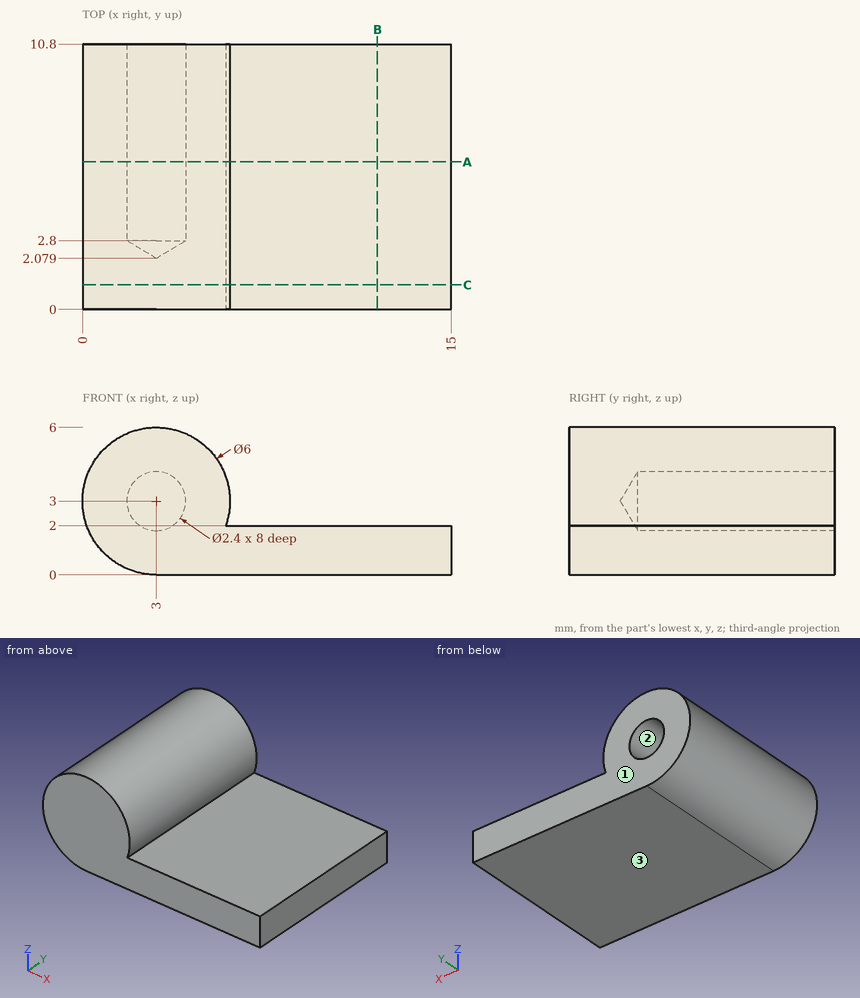
Design review of the part shown in the three views and the two pictorial views. Dimensions are in mm from the part's minimum x, y and z. Round coordinates to 2 decimals unless told otherwise and drop trailing zeros. Order: outer loops, then holes, each group sorted by start corner. A loop starts at its lowest first (then second) coordinate and runs counter-clockwise, first axis right, second up. Notation, with made-up numbers: (-19, -34.5) -> (17, -34.5) arc R21 cw to (17, -29.5) -> close; hole circle Ø9 at (14, 39). An arc over 180 degrees is marked (long way). Write item = value, one per line. Start each with the question number.
1) Take a section at B-B on x = 12. State the section outline as (y, z) points.
2) The part is to be moulded in two halves that separate along Z. For the marked faces 1, 2 and 3, say which applies: +Z half, -Z half, draft (parallel to the pull), parting line (faces both ways), or undercut.
3) To check wall thickness, follow line 1 (X direction, y = 9, z = 3); line 2 (Z direction, x = 13.25, y = 1); line 3 (Z direction, x = 3.5, y = 2.5). State the ranges of each line that lie inside material, in increasing order. Write a range as from..to.
4) Take a section at A-A on y = 6. State the section outline as (x, z) points, plus the area to 3 significant figures.
5) Take a section at C-C on y = 1. State the section outline as (x, z) points, plus the area to 4 significant figures.
6) Insertion check: pin 1 (1.5 mm diameter, centred on y = 6.5, z = 2, fed in from -X); pin 2 (1.4 mm diameter, centred on x = 3, z = 3, fed in from +Y); pin 3 (4 mm diameter, centred on x = 8.5, y = 9.5, fed in from +Z). Each pin has a flat end and moves straight along its axis. Give the tip position at first contact, or say it passes through.
Verdict:
q1.outline = (0, 0) -> (10.8, 0) -> (10.8, 2) -> (0, 2) -> close
q2.face_1 = draft
q2.face_2 = undercut
q2.face_3 = -Z half
q3.line_1 = 0..1.8, 4.2..6
q3.line_2 = 0..2
q3.line_3 = 0..2.51, 3.49..5.96
q4.outline = (3, 0) -> (15, 0) -> (15, 2) -> (5.83, 2) arc R3 ccw (long way) to start; hole circle Ø2.4 at (3, 3)
q4.area = 43.6 mm2
q5.outline = (3, 0) -> (15, 0) -> (15, 2) -> (5.83, 2) arc R3 ccw (long way) to start
q5.area = 48.15 mm2
q6.pin_1 = 0.01
q6.pin_2 = 2.5
q6.pin_3 = 2
